Geometry check sheet. Reference: the model listing, model coordinates, mm. Give positions to 0.01 mm unless a question says otherwise; leave off trailing zeros. Loops run counter-clockwise (first coordinate to the right, second up) from the corner with the lowest first, then second, coordinate; pieces in that order, holes last.
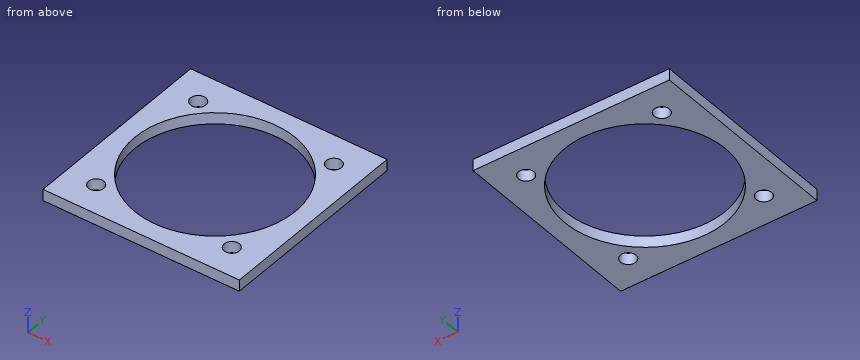
```python
from build123d import *

# Parameters (mm, degrees)
SKETCH1_W           = 55
SKETCH1_H           = 55
SKETCH1_R           = 22.5
SKETCH1_R_2         = 2.15
BOSS_EXTRUDE1_DEPTH = 3.175


with BuildPart() as part:
    # Sketch1 → Boss-Extrude1 (new body)
    with BuildSketch(Plane.XY):
        Rectangle(SKETCH1_W, SKETCH1_H)
        with Locations(Location((0, 0, 0), (0, 0, 180))):
            Circle(SKETCH1_R, mode=Mode.SUBTRACT)
        with Locations(Location((19, 19, 0), (0, 0, 180))):
            Circle(SKETCH1_R_2, mode=Mode.SUBTRACT)
        with Locations(Location((19, -19, 0), (0, 0, 180))):
            Circle(SKETCH1_R_2, mode=Mode.SUBTRACT)
        with Locations(Location((-19, -19, 0), (0, 0, 180))):
            Circle(SKETCH1_R_2, mode=Mode.SUBTRACT)
        with Locations(Location((-19, 19, 0), (0, 0, 180))):
            Circle(SKETCH1_R_2, mode=Mode.SUBTRACT)
    extrude(amount=BOSS_EXTRUDE1_DEPTH)


solid = part.part
```
1) Sectioned sample at A-A on y = 0. Enter the section's corners in (x, z) (3 decimals), plus the area to 4 significant figures.
2) Scan lines: line 1 along Y through (x, z) = (0, 1.95); line 2 along X through (y, z) = (20, 1.1); line 3 along Y through (x, z) = (-18, 1.35). Record each from-to range of solid material in increasing order.
3) Depth check by flat-ended pin: P1, Ø5, axis at x = 19, y = 19, coming from the +Z side (3 decimals). Enter the tip coordinate at first touch or a pass-through.
4) Sectioned sample at C-C on z = 1.9. Enter the section's corners in (x, y), plus the area to 3 significant figures.
5) Sectioned sample at B-B on x = 19. Enter the section's corners in (y, z) (3 decimals).
Determined:
1. outline: (-27.5, 0) - (-22.5, 0) - (-22.5, 3.175) - (-27.5, 3.175) - close; (22.5, 0) - (27.5, 0) - (27.5, 3.175) - (22.5, 3.175) - close
1. area: 31.75 mm2
2. line 1: y = -27.5 to -22.5, 22.5 to 27.5
2. line 2: x = -27.5 to -20.9, -17.1 to -10.31, 10.31 to 17.1, 20.9 to 27.5
2. line 3: y = -27.5 to -20.9, -17.1 to -13.5, 13.5 to 17.1, 20.9 to 27.5
3. P1: stops at z = 3.175
4. outline: (-27.5, -27.5) - (27.5, -27.5) - (27.5, 27.5) - (-27.5, 27.5) - close; hole circle Ø45 at (0, 0); hole circle Ø4.3 at (-19, -19); hole circle Ø4.3 at (-19, 19); hole circle Ø4.3 at (19, -19); hole circle Ø4.3 at (19, 19)
4. area: 1,380 mm2
5. outline: (-27.5, 0) - (-21.15, 0) - (-21.15, 3.175) - (-27.5, 3.175) - close; (-16.85, 0) - (-12.052, 0) - (-12.052, 3.175) - (-16.85, 3.175) - close; (12.052, 0) - (16.85, 0) - (16.85, 3.175) - (12.052, 3.175) - close; (21.15, 0) - (27.5, 0) - (27.5, 3.175) - (21.15, 3.175) - close
